Work out the finished part from the listing and answer in its coordinate system (mm). Face numbers are marked on the shaded views. A direction names the side the tool comes from. Round coordinates to 2 decimals unless told otherwise and drop trailing zeros. Order: outer loops, then holes, each group sorted by start corner. A loop starts at its lowest first (then second) coordinate and runs counter-clockwise, first axis right, second up. Notation, with made-up numbers: M -9.75,-17 L 46.25,-17 A7 ccw 46.25,-5 Z; hole C -34.5,62.5 d5. An arc over 180 degrees is marked long. Return JSON: item names as keys, results as strings.
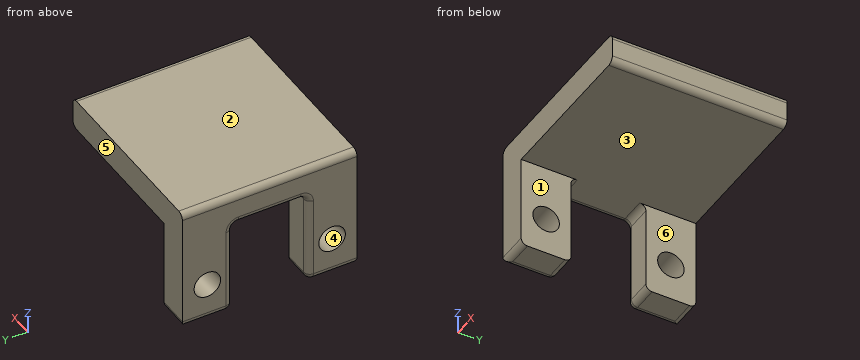
from build123d import *

# Parameters (mm, degrees)
SKETCH1_W           = 25
SKETCH1_H           = 5
BOSS_EXTRUDE1_DEPTH = 28
BOSS_EXTRUDE3_DEPTH = 5
FILLET2_R           = 1
CUT_EXTRUDE2_REACH  = 46.612
SKETCH5_R           = 2.125


with BuildPart() as part:
    # Sketch1 → Boss-Extrude1 (new body)
    with BuildSketch(Plane(origin=(0, 0, 0), x_dir=(1, 0, 0), z_dir=(0, 1, 0))):
        Rectangle(SKETCH1_W, SKETCH1_H)
    extrude(amount=BOSS_EXTRUDE1_DEPTH)

    # Sketch4 → Boss-Extrude3 (add)
    with BuildSketch(Plane.ZY.offset(12.5)):
        Polygon((-17.5, 20), (-2.5, 20), (-2.5, 8), (-17.5, 8), (-17.5, 0), (2.5, 0), (2.5, 28), (-17.5, 28), align=None)
    extrude(amount=BOSS_EXTRUDE3_DEPTH)

    # Fillet2
    fillet2_edges = [part.edges().sort_by_distance(p)[0] for p in [
        (-15, 28, -17.5),
        (-15, 20, -17.5),
        (-15, 20, -2.5),
        (-15, 8, -2.5),
        (-15, 8, -17.5),
        (-15, 0, -17.5),
        (-17.5, 14, 2.5),
        (-17.5, 24, -17.5),
        (-17.5, 20, -10),
        (-17.5, 14, -2.5),
        (-17.5, 8, -10),
        (-17.5, 4, -17.5),
        (12.5, 14, 2.5),
        (12.5, 14, -2.5),
    ]]
    fillet(fillet2_edges, radius=FILLET2_R)

    # Sketch5 → Cut-Extrude2 (cut, up to next)
    with BuildSketch(Plane.ZY.offset(17.5), mode=Mode.PRIVATE) as cut_extrude2_sk1:
        with Locations((-11.5, 24)):
            Circle(SKETCH5_R)
    cut_extrude2_tool1 = extrude(cut_extrude2_sk1.sketch, amount=-CUT_EXTRUDE2_REACH, mode=Mode.PRIVATE) & part.part
    # Sketch5 → Cut-Extrude2 (cut, up to next)
    with BuildSketch(Plane.ZY.offset(17.5), mode=Mode.PRIVATE) as cut_extrude2_sk2:
        with Locations((-11.5, 4)):
            Circle(SKETCH5_R)
    cut_extrude2_tool2 = extrude(cut_extrude2_sk2.sketch, amount=-CUT_EXTRUDE2_REACH, mode=Mode.PRIVATE) & part.part
    add(cut_extrude2_tool1.solids().sort_by_distance((-17.5, 24, -11.5))[0], mode=Mode.SUBTRACT)
    add(cut_extrude2_tool2.solids().sort_by_distance((-17.5, 4, -11.5))[0], mode=Mode.SUBTRACT)


solid = part.part
Item 1: Find section A-A (z = -4). Determine the outline of the cut face in (x, y).
Output:
{"outline": "M -17.5,0 L -12.5,0 L -12.5,8 L -16.5,8 A1 ccw -17.5,7 Z; M -17.5,21 A1 ccw -16.5,20 L -12.5,20 L -12.5,28 L -17.5,28 Z"}
Item 2: Find section C-C (z = -11.5). Determine the outline of the cut face in (x, y) (3 decimals), plus the area to 3 significant figures.
Output:
{"outline": "M -17.5,0 L -12.5,0 L -12.5,1.875 L -17.5,1.875 Z; M -17.5,6.125 L -12.5,6.125 L -12.5,8 L -16.5,8 A1 ccw -17.5,7 Z; M -17.5,21 A1 ccw -16.5,20 L -12.5,20 L -12.5,21.875 L -17.5,21.875 Z; M -17.5,26.125 L -12.5,26.125 L -12.5,28 L -17.5,28 Z", "area": "37.1 mm^2"}
Item 3: Find section B-B (y = 4). Determine the outline of the cut face in (x, z) (3 decimals), plus the area to 3 significant figures.
Output:
{"outline": "M -17.5,-16.5 A1 ccw -16.5,-17.5 L -12.5,-17.5 L -12.5,-13.625 L -17.5,-13.625 Z; M -17.5,-9.375 L -12.5,-9.375 L -12.5,-2.5 L 11.5,-2.5 A1 ccw 12.5,-1.5 L 12.5,1.5 A1 ccw 11.5,2.5 L -16.5,2.5 A1 ccw -17.5,1.5 Z", "area": "203 mm^2"}
Item 4: Each of these flat-tipped pins is pushed along its axis until it touches: pin 1 (3 mm diameter, centred on y = 9, z = -6, fed in from -X); pin 2 (2.5 mm diameter, centred on y = 5.5, z = -13, fed in from +X); pin 3 (1.5 mm diameter, centred on y = 4, z = -10.5, fed in from +X); pin 4 (8 mm diameter, centred on x = -6.5, y = 11.5, fed in from -Z). Where does it stop, or does it pass through?
Output:
{"pin 1": "stops at x = -17.37", "pin 2": "stops at x = -12.5", "pin 3": "passes through", "pin 4": "stops at z = -2.5"}
Item 5: Consider line 1 along Y through (x, z) = (-14.6, -11.5) (3 decimals); line 2 along Y through (x, z) = (-16, -5.75); line 3 along Z through (x, y) = (8, 15.25). Determine where each line is inside the solid, lowest interval first. Write a range as [from, to].
Output:
{"line 1": "y = [0, 1.875], [6.125, 8], [20, 21.875], [26.125, 28]", "line 2": "y = [0, 8], [20, 28]", "line 3": "z = [-2.5, 2.5]"}
Item 6: Find section D-D (y = 16.5). Determine the outline of the cut face in (x, z).
Output:
{"outline": "M -17.5,-1.5 A1 ccw -16.5,-2.5 L 11.5,-2.5 A1 ccw 12.5,-1.5 L 12.5,1.5 A1 ccw 11.5,2.5 L -16.5,2.5 A1 ccw -17.5,1.5 Z"}
Item 7: The mould has two halves that part along Z. Classify the marked faces 1, 2, 3 and 4: pulls with the +Z half, pulls with the -Z half, needs draft (parallel to the pull), parting line crosses it, or undercut.
Output:
{"face 1": "needs draft", "face 2": "pulls with the +Z half", "face 3": "pulls with the -Z half", "face 4": "undercut"}
Item 8: Which of the six approach directions +Z, -Z, +X, -X, +Y, -Y give full straight-line access (tool end or side, diameter ignored) to the marked faces 5 and 6?
Output:
{"face 5": "+Z, -Z, +X, -X, +Y", "face 6": "-Z, +X, +Y, -Y"}
